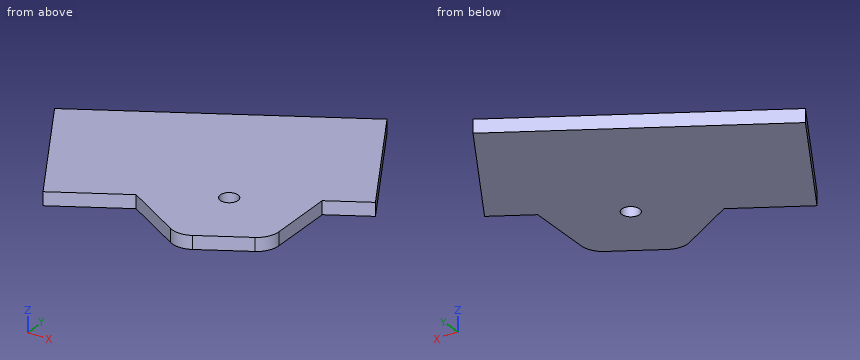
```python
from build123d import *

# Parameters (mm, degrees)
SKETCH1_R           = 4
BOSS_EXTRUDE1_DEPTH = 6


with BuildPart() as part:
    # Sketch1 → Boss-Extrude1 (new body)
    with BuildSketch(Plane.XY):
        with BuildLine():
            Line((95.687041803, 386.103563742), (62.675802399, 442.096939002))
            Line((62.675802399, 442.096939002), (-45.003765409, 378.613786303))
            Line((-45.003765409, 378.613786303), (-11.992526005, 322.620411043))
            Line((-11.992526005, 322.620411043), (18.157752981, 340.395693799))
            Line((18.157752981, 340.395693799), (43.600659694, 326.013529743))
            ThreePointArc((43.600659694, 326.013529743), (48.612652005, 324.719368889), (53.600245097, 326.104588867))
            Line((53.600245097, 326.104588867), (73.80351169, 338.015549175))
            ThreePointArc((73.80351169, 338.015549175), (77.430284022, 341.708981412), (78.724444877, 346.720973723))
            Line((78.724444877, 346.720973723), (78.458310954, 375.94625931))
            Line((78.458310954, 375.94625931), (95.687041803, 386.103563742))
        make_face()
        with Locations((48.308031967, 358.170976554)):
            Circle(SKETCH1_R, mode=Mode.SUBTRACT)
    extrude(amount=BOSS_EXTRUDE1_DEPTH)


solid = part.part
```
The listing builds one solid part. Answer for the finished solid, in the listing's coordinates (mm). Round coordinates to 2 decimals unless told otherwise and drop trailing zeros. Write each loop counter-clockwise with the first axis right and the second up, starting at its lowest first coordinate (ties: lowest second). Pieces come first, ordered by that corner, then holes. Notation, with made-up numbers: (-8.5, 58) -> (0.5, 58) arc R20 ccw to (0.5, 82) -> close; hole circle Ø4 at (6, -14). An arc over 180 degrees is marked (long way). Answer as a JSON object with one key per item and string values. Group by question number.
Q1. Section B-B (y = 330) is taken. Write down the section's boundary in (x, z).
Q2. Section C-C (x = 72) is taken. Write down the section's boundary in (y, z).
Q3. Straight lines are drawn through the part: line 1 along Y through (x, z) = (-23.5, 5.3); line 2 along Y through (x, z) = (-18, 4.7); line 3 along X through (y, z) = (351.5, 3.75). For each, find the intervals that lie inside material, in ascending order.
Q4. Section D-D (y = 421) is taken. Write down the section's boundary in (x, z), plus the area to 3 significant figures.
Q5. Each of these flat-tipped pins is pushed along its axis until it touches: pin 1 Ø1 at (x, z) = (54, 0.5) entering from -Y; pin 2 Ø3 at (x, z) = (34.5, 5) entering from +Y; pin 3 Ø2 at (x, z) = (71.5, 4.5) entering from -Y. Where does it stop, or does it pass through?
Q6. Section A-A (z = 1.3) is taken. Write down the section's boundary in (x, y).
Check values:
{
 "1": {"outline": "(-16.34, 0) -> (0.52, 0) -> (0.52, 6) -> (-16.34, 6) -> close; (36.55, 0) -> (60.21, 0) -> (60.21, 6) -> (36.55, 6) -> close"},
 "2": {"outline": "(336.95, 0) -> (426.28, 0) -> (426.28, 6) -> (336.95, 6) -> close"},
 "3": {"line 1": "342.14 to 391.29", "line 2": "332.81 to 394.53", "line 3": "-29.02 to 78.68"},
 "4": {"outline": "(26.89, 0) -> (75.11, 0) -> (75.11, 6) -> (26.89, 6) -> close", "area": "289 mm^2"},
 "5": {"pin 1": "y = 326.05", "pin 2": "y = 426.37", "pin 3": "y = 336.07"},
 "6": {"outline": "(-45, 378.61) -> (-11.99, 322.62) -> (18.16, 340.4) -> (43.6, 326.01) arc R10 ccw to (53.6, 326.1) -> (73.8, 338.02) arc R10 ccw to (78.72, 346.72) -> (78.46, 375.95) -> (95.69, 386.1) -> (62.68, 442.1) -> close; hole circle Ø8 at (48.31, 358.17)"}
}
